Autodesk Inventor part; units mm, degrees
ref_plane "YZ Plane" through (0, 0, 0) normal (1, 0, 0) x (0, 1, 0)
ref_plane "XZ Plane" through (0, 0, 0) normal (0, 1, 0) x (-1, 0, 0)
ref_plane "XY Plane" through (0, 0, 0) normal (0, 0, 1) x (1, 0, 0)
sketch "Sketch1" plane through (0, 0, 0) normal (0, 0, 1) x (1, 0, 0)
  circle A0 centre (0, 0) radius 38.75
  dimension "d0" = 77.5
extrude "Extrusion1" add sketch "Sketch1" along normal blind 165.1
sketch "Sketch2" plane through (0, 0, 165.1) normal (0, 0, 1) x (1, 0, 0)
  line L0 (-27.305, -2.5) -> (27.305, -2.5)
  line L1 (27.305, -2.5) -> (27.305, 2.5)
  line L2 (27.305, 2.5) -> (-27.305, 2.5)
  line L3 (-27.305, 2.5) -> (-27.305, -2.5)
  line L4 (-27.305, -2.5) -> (27.305, 2.5) construction
  line L5 (27.305, -2.5) -> (-27.305, 2.5) construction
  line L6 (0, 2.5) -> (41.5863, 2.5)
  line L7 (41.5863, 2.5) -> (41.5863, 42.5)
  line L8 (41.5863, 42.5) -> (0, 42.5)
  line L9 (0, 42.5) -> (0, 2.5)
  line L10 (0, 42.5) -> (-50, 42.5)
  line L11 (-50, 42.5) -> (-50, 2.5)
  line L12 (-50, 2.5) -> (0, 2.5)
  line L13 (0, 2.5) -> (0, 42.5)
  point P0 (0, 0)
  point P1 (-27.305, 2.5)
  dimension "d3" = 54.61
  dimension "d4" = 5
extrude "Extrusion2" cut sketch "Sketch2" against normal through all
sketch "Sketch3" plane through (0, 0, 0) normal (0, 0, -1) x (-1, 0, 0)
  circle A0 centre (0, 0) radius 42
extrude "Extrusion3" add sketch "Sketch3" along normal blind 2
sketch "Sketch4" plane through (-27.305, -2.5, 165.1) normal (0, 1, 0) x (1, 0, 0)
  line L0 (0, 165.1) -> (54.61, 165.1)
  line L1 (0, 0) -> (0, 165.1)
  point P0 (27.305, 165.1)
  point P1 (27.305, 158.496)
  dimension "d9" = 6.604
  dimension "d10" = 27.305
hole "Hole1" at (0, -2.5, 6.604) direction (0, -1, 0) diameter 2.6416 depth 10.979
sketch "Sketch5" plane through (-27.305, -2.5, 165.1) normal (0, 1, 0) x (1, 0, 0)
  line L0 (0, 165.1) -> (54.61, 165.1)
  line L1 (0, 0) -> (0, 165.1)
  point P0 (27.305, 165.1)
  point P1 (27.305, 80.01)
  dimension "d18" = 85.09
  dimension "d26" = 27.305
hole "Hole2" at (0, -2.5, 85.09) direction (0, -1, 0) diameter 2.6416 depth 10.979
shell "Shell1" thickness 2 removed faces 1 at (1.4054, -14.5066, 165.1)
sketch "Sketch6" plane through (27.305, 2.5, 165.1) normal (0, 1, 0) x (1, 0, 0)
  circle A0 centre (-27.305, 158.496) radius 1.3208
  circle A1 centre (-27.305, 80.01) radius 1.3208
  line L0 (0, 79.02) -> (0, 81)
  line L1 (-54.61, 81) -> (-54.61, 79.02)
  line L2 (0, 160.401) -> (0, 156.591)
  line L3 (-54.61, 156.591) -> (-54.61, 160.401)
  line L4 (-54.61, 160.401) -> (0, 156.591) construction
  line L5 (0, 160.401) -> (-54.61, 156.591) construction
  line L6 (0, 78.105) -> (0, 81.915)
  line L7 (-54.61, 81.915) -> (-54.61, 78.105)
  line L8 (-54.61, 78.105) -> (0, 81.915) construction
  line L9 (0, 78.105) -> (-54.61, 81.915) construction
  line L10 (-54.61, 165.1) -> (0, 165.1)
  line L11 (0, 165.1) -> (0, 0)
  line L12 (0, 0) -> (-54.61, 0)
  line L13 (-54.61, 0) -> (-54.61, 165.1)
  arc A2 (-25.1118, 160.401) -> (-29.4982, 160.401) centre (-27.305, 158.496) ccw
  arc A3 (-29.4982, 156.591) -> (-25.1118, 156.591) centre (-27.305, 158.496) ccw
  line L14 (-54.61, 160.401) -> (-29.4982, 160.401)
  line L15 (-25.1118, 160.401) -> (0, 160.401)
  line L16 (0, 156.591) -> (-25.1118, 156.591)
  line L17 (-29.4982, 156.591) -> (-54.61, 156.591)
  line L18 (0, 81.915) -> (-25.1118, 81.915)
  line L19 (-29.4982, 81.915) -> (-54.61, 81.915)
  line L20 (-54.61, 78.105) -> (-29.4982, 78.105)
  line L21 (-25.1118, 78.105) -> (0, 78.105)
  arc A4 (-25.1118, 81.915) -> (-29.4982, 81.915) centre (-27.305, 80.01) ccw
  arc A5 (-29.4982, 78.105) -> (-25.1118, 78.105) centre (-27.305, 80.01) ccw
  point P0 (-27.305, 165.1)
extrude "Extrusion4" cut sketch "Sketch6" against normal blind 12.5 contours L11 L12 L13 L20 A5 L21 | L18 A4 L19 L13 L17 A3 L16 L11 | L15 A2 L14 L13 L10 L11
sketch "Sketch7" plane through (0, 0, 0) normal (1, 0, 0) x (0, 1, 0)
  line L0 (-4.5, 165.1) -> (-4.5, 0)
  line L1 (-4.5, 0) -> (-49, 0)
  line L2 (0.5, 0) -> (-4.5, 0)
  line L3 (-4.5, 0) -> (-55.1519, 0)
  line L4 (-55.1519, 0) -> (-55.1519, 156.9376)
  line L5 (-55.1519, 156.9376) -> (-4.5, 156.9376)
  line L6 (-4.5, 156.9376) -> (-4.5, 0)
  line L7 (-4.5, 0) -> (-56.1519, 0)
  line L8 (-56.1519, 0) -> (-56.1519, 0)
  line L9 (-56.1519, 0) -> (-4.5, 0)
  line L10 (-4.5, 0) -> (-4.5, 0)
  point P0 (0, 0)
  point P1 (-4.5, 156.9376)
  point P2 (-55.1519, 1)
  point P3 (-4.5, 0)
extrude "Extrusion5" cut sketch "Sketch7" along normal through all both and the other way through all
sketch "Sketch9" plane through (0, 0, 0) normal (0, 0, 1) x (1, 0, 0)
  line L0 (-27.305, -4.5) -> (-27.305, 2.5)
  line L1 (-27.305, -1) -> (-27.305, 7.524)
  line L2 (-27.305, -4.5) -> (-27.305, -7.524)
  line L3 (27.305, 2.5) -> (27.305, -4.5)
  line L4 (27.305, -1) -> (27.305, 7.524)
  line L5 (27.305, 7.524) -> (27.305, -7.524)
  arc A0 (-27.305, -7.524) -> (27.305, -7.524) centre (0, 0) ccw
  arc A1 (27.305, 7.524) -> (-27.305, 7.524) centre (0, 0) ccw
  point P0 (-27.305, 2.5)
extrude "Extrusion7" cut sketch "Sketch9" against normal blind 2.5
sketch "Sketch14" plane through (2.1932, -2.5, 86.995) normal (0, 1, 0) x (1, 0, 0)
  circle A0 centre (-2.1932, 80.391) radius 1.3208
  circle A1 centre (-2.1932, 80.391) radius 1.3208
  circle A2 centre (-2.1932, 80.391) radius 2.905
  circle A3 centre (-2.1932, 1.905) radius 1.3208
  circle A4 centre (-2.1932, 1.905) radius 1.3208
  circle A5 centre (-2.1932, 1.905) radius 2.905
  point P0 (-2.1932, 86.995)
extrude "Extrusion10" add sketch "Sketch14" along normal blind 2
properties part number "Revised Mount"
Can you work these out from the model? Positions are in its coordinate system, mm. A direction names the side the tool comes from. Coordinates: 2 decimals unless noted, no trailing zeros. Loops run counter-clockwise (first coordinate to the right, second up) from the corner with the lowest first, then second, coordinate; pieces in that order, holes last.
Item 1: Please list where these lines run through material, in increasing order: L1, parallel to Z at x = 0, y = -2 (3 decimals); L2, parallel to X at y = 0, z = 26 (3 decimals); L3, parallel to Z at x = 36, y = 15.5.
Answers below:
L1: z = 3.699 to 5.283, 7.925 to 9.509, 82.185 to 83.769, 86.411 to 87.995
L2: x = -38.75 to -36.75, -29.305 to -27.305, 27.305 to 29.305, 36.75 to 38.75
L3: z = -2 to 0
Item 2: If we mould it in two halves opening along Z, with no side actions, what happens to faces 1 (the face through (-27.4, -8.7, -2)), 2 (the face through (0, -37, 156.938)), 3 (the face through (-0.38, -1.51, 87.97)), 4 (the face through (0.516, 28.318, -0.986))? For each: released by +Z, released by -Z, zero draft, split by the parting line, or undercut.
Answers below:
face 1: released by -Z
face 2: undercut
face 3: undercut
face 4: zero draft
Item 3: I'm going to push flat-ended pins straight in: pin 1 (2.5 mm diameter, centred on x = 0, z = 85.09, fed in from -Y); pin 2 (1.5 mm diameter, centred on x = -4.5, y = -2, fed in from +Z) (3 decimals); pin 3 (1.9 mm diameter, centred on x = -12.5, z = 6.5, fed in from +Y); pin 4 (1.7 mm diameter, centred on x = -1, z = 8, fed in from +Y). Where does each tip first touch, or does it pass through?
Answers below:
pin 1: passes through
pin 2: stops at z = 86.995
pin 3: stops at y = -2.5
pin 4: stops at y = -0.5
Item 4: Which directions (+Z, -Z, +X, -X, +Y, -Y) give clear straight access to the entire face, cutting with the end or side of a thin tool? Please do faces 5 (the face through (-0.63, -1.51, 3.77)), 6 (the face through (-33, 2.5, 84)), 7 (the face through (1, -0.5, 8)), 8 (the face through (-36.7, -1.9, 106.6)).
Answers below:
face 5: +Y
face 6: +Z, +X, -X, +Y
face 7: +Z, -Z, +Y
face 8: +Z
Item 5: Suppose I cut it at A-A (y = 12). Please give me the cut outline in (x, z).
Answers below:
outline: (-40.25, -2) - (-25.65, -2) - (-25.65, 0) - (-40.25, 0) - close; (25.65, -2) - (40.25, -2) - (40.25, 0) - (25.65, 0) - close
Item 6: Suppose I cut it at B-B (z = 130.5). Please give me the cut outline in (x, y) (3 decimals), then the cut area to 3 significant figures.
Answers below:
outline: (-38.669, 2.5) arc R38.75 ccw to (-38.488, -4.5) - (-36.473, -4.5) arc R36.75 cw to (-36.747, 0.5) - (-29.305, 0.5) - (-29.305, -4.5) - (-27.305, -4.5) - (-27.305, 2.5) - close; (27.305, -4.5) - (29.305, -4.5) - (29.305, 0.5) - (36.747, 0.5) arc R36.75 cw to (36.473, -4.5) - (38.488, -4.5) arc R38.75 ccw to (38.669, 2.5) - (27.305, 2.5) - close
area: 85.7 mm2
Item 7: Suppose I cut it at C-C (x = -14.5). Please give me the cut outline in (y, z) (3 decimals).
Answers below:
outline: (-39.418, -2) - (-24.329, -2) - (-24.329, 0) - (-39.418, 0) - close; (-35.935, 156.938) - (-33.769, 156.938) - (-33.769, 165.1) - (-35.935, 165.1) - close; (-4.5, 4.699) - (-2.5, 4.699) - (-2.5, 8.509) - (-4.5, 8.509) - close; (-4.5, 83.185) - (-2.5, 83.185) - (-2.5, 86.995) - (-4.5, 86.995) - close; (24.329, -2) - (39.418, -2) - (39.418, 0) - (24.329, 0) - close
Item 8: Suppose I cut it at D-D (y = -34). Please give me the cut outline in (x, z), then the cut area to 3 significant figures.
Answers below:
outline: (-24.66, -2) - (24.66, -2) - (24.66, 0) - (-24.66, 0) - close; (-18.59, 156.94) - (-13.95, 156.94) - (-13.95, 165.1) - (-18.59, 165.1) - close; (13.95, 156.94) - (18.59, 156.94) - (18.59, 165.1) - (13.95, 165.1) - close
area: 174 mm2
